Build history of the part. All positions in model axes, mm. A direction names the side the tool comes from. Round coordinates to 2 decimals unless told otherwise and drop trailing zeros. Write each loop counter-clockwise with the first axis right and the second up, starting at its lowest first coordinate (ties: lowest second). Pieces come first, ordered by that corner, then holes. Notation, with made-up numbers: (-32, 16.25) - (26, 16.25) arc R32 ccw to (26, 44.25) - close; hole circle Ø8 at (39.25, 80.25). An arc over 180 degrees is marked (long way). Write each question's results on one line, items separated by ' | '.
from build123d import *

# Parameters (mm, degrees)
EXTRUDE_1_DEPTH     = 3
SKETCH_2_W          = 40.5
SKETCH_2_H          = 13.3
SKETCH_2_W_2        = 20
SKETCH_2_H_2        = 9
SKETCH_2_W_3        = 14
SKETCH_2_H_3        = 20
SKETCH_2_W_4        = 29
SKETCH_2_H_4        = 32
CUT_EXTRUDE_1_DEPTH = 3
SKETCH_3_W          = 51.3
SKETCH_3_H          = 3
CUT_EXTRUDE_2_DEPTH = 3
SKETCH_4_W          = 4
SKETCH_4_H          = 28
SKETCH_4_W_2        = 14
SKETCH_4_H_2        = 14
EXTRUDE_2_DEPTH     = 14
CUT_EXTRUDE_3_DEPTH = 14
CUT_EXTRUDE_4_DEPTH = 14
CUT_EXTRUDE_5_DEPTH = 14
CUT_EXTRUDE_6_REACH = 216.55
SKETCH_9_R          = 2.5


with BuildPart() as part:
    # Эскиз1 → Бобышка-Вытянуть1 (new body)
    with BuildSketch(Plane(origin=(0, 0, 0), x_dir=(1, 0, 0), z_dir=(0, 1, 0))):
        Polygon((-121.424018304, 15.144551695), (-121.424018304, 41.394551695), (183.575981696, 41.394551695), (183.575981696, 15.144551695), (186.575981696, 15.144551695), (186.575981696, -11.105448305), (183.575981696, -11.105448305), (183.575981696, -37.355448305), (186.575981696, -37.355448305), (186.575981696, -63.605448305), (-118.424018304, -63.605448305), (-118.424018304, -37.355448305), (-121.424018304, -37.355448305), (-121.424018304, -11.105448305), (-118.424018304, -11.105448305), (-118.424018304, 15.144551695), align=None)
    extrude(amount=EXTRUDE_1_DEPTH)

    # Эскиз2 → Вырез-Вытянуть1 (cut)
    with BuildSketch(Plane(origin=(0, 3, 0), x_dir=(1, 0, 0), z_dir=(0, 1, 0))):
        with Locations((-58.674018304, -36.955448305)):
            Rectangle(SKETCH_2_W, SKETCH_2_H)
        with Locations((-6.874018304, -36.955448305)):
            Rectangle(SKETCH_2_W, SKETCH_2_H)
        with Locations((-6.874018304, -20.355448305)):
            Rectangle(SKETCH_2_W, SKETCH_2_H)
        with Locations((-58.674018304, -20.355448305)):
            Rectangle(SKETCH_2_W, SKETCH_2_H)
        with Locations((-6.874018304, -3.755448305)):
            Rectangle(SKETCH_2_W, SKETCH_2_H)
        with Locations((48.575981696, -1.605448305)):
            Rectangle(SKETCH_2_W_2, SKETCH_2_H_2)
        with Locations((105.575981696, -7.105448305)):
            Rectangle(SKETCH_2_W_3, SKETCH_2_H_3)
        with Locations((147.075981696, -13.105448305)):
            Rectangle(SKETCH_2_W_4, SKETCH_2_H_4)
    extrude(amount=-CUT_EXTRUDE_1_DEPTH, mode=Mode.SUBTRACT)

    # Эскиз3 → Вырез-Вытянуть2 (cut)
    with BuildSketch(Plane(origin=(0, 3, 0), x_dir=(1, 0, 0), z_dir=(0, 1, 0))):
        with Locations((-95.774018304, -62.105448305)):
            Rectangle(SKETCH_3_W, SKETCH_3_H)
        with Locations((6.825981696, -62.105448305)):
            Rectangle(SKETCH_3_W, SKETCH_3_H)
        with Locations((109.425981696, -62.105448305)):
            Rectangle(SKETCH_3_W, SKETCH_3_H)
    extrude(amount=-CUT_EXTRUDE_2_DEPTH, mode=Mode.SUBTRACT)

    # Эскиз4 → Бобышка-Вытянуть2 (add)
    with BuildSketch(Plane.XZ):
        with Locations((27.575981696, -27.394551695)):
            Rectangle(SKETCH_4_W, SKETCH_4_H)
        with Locations((-111.424018304, -34.394551695)):
            Rectangle(SKETCH_4_W_2, SKETCH_4_H_2)
        with Locations((176.575981696, -34.394551695)):
            Rectangle(SKETCH_4_W_2, SKETCH_4_H_2)
        with Locations((37.575981696, -27.394551695)):
            Rectangle(SKETCH_4_W, SKETCH_4_H)
    extrude(amount=EXTRUDE_2_DEPTH)

    # Эскиз6 → Вырез-Вытянуть3 (cut)
    with BuildSketch(Plane(origin=(39.575981696, 0, 0), x_dir=(0, 0, -1), z_dir=(1, 0, 0))):
        Polygon((13.394551695, -14), (13.394551695, 0), (38.394551695, -14), align=None)
    extrude(amount=-CUT_EXTRUDE_3_DEPTH, mode=Mode.SUBTRACT)

    # Эскиз7 → Вырез-Вытянуть4 (cut)
    with BuildSketch(Plane(origin=(183.575981696, 0, 0), x_dir=(0, 0, -1), z_dir=(1, 0, 0))):
        Polygon((27.394551695, -14), (27.394551695, 0), (38.394551695, -14), align=None)
    extrude(amount=-CUT_EXTRUDE_4_DEPTH, mode=Mode.SUBTRACT)

    # Эскиз8 → Вырез-Вытянуть5 (cut)
    with BuildSketch(Plane(origin=(-104.424018304, 0, 0), x_dir=(0, 0, -1), z_dir=(1, 0, 0))):
        Polygon((27.394551695, -14), (27.394551695, 0), (38.394551695, -14), align=None)
    extrude(amount=-CUT_EXTRUDE_5_DEPTH, mode=Mode.SUBTRACT)

    # Вырез-Вытянуть6: up to this plane
    cut_extrude_6_end = Plane(origin=(169.575981696, -14, -38.394551695), z_dir=(0, 0.6178215519319037, -0.7863183388224225))
    # Эскиз9 → Вырез-Вытянуть6 (cut, up to the surface)
    with BuildSketch(Plane(origin=(0, 0, -41.394551695), x_dir=(-1, 0, 0), z_dir=(0, 0, -1)), mode=Mode.PRIVATE) as cut_extrude_6_sk1:
        with Locations((-176.575981696, -7)):
            Circle(SKETCH_9_R)
    cut_extrude_6_tool1 = split(extrude(cut_extrude_6_sk1.sketch, amount=-CUT_EXTRUDE_6_REACH, mode=Mode.PRIVATE), bisect_by=cut_extrude_6_end, keep=Keep.BOTH, mode=Mode.PRIVATE)
    add(cut_extrude_6_tool1.solids().sort_by_distance((176.575982, -7, -41.394552))[0], mode=Mode.SUBTRACT)
    # Эскиз9 → Вырез-Вытянуть6 (cut, up to the surface)
    with BuildSketch(Plane(origin=(0, 0, -41.394551695), x_dir=(-1, 0, 0), z_dir=(0, 0, -1)), mode=Mode.PRIVATE) as cut_extrude_6_sk2:
        with Locations((111.424018304, -7)):
            Circle(SKETCH_9_R)
    cut_extrude_6_tool2 = split(extrude(cut_extrude_6_sk2.sketch, amount=-CUT_EXTRUDE_6_REACH, mode=Mode.PRIVATE), bisect_by=cut_extrude_6_end, keep=Keep.BOTH, mode=Mode.PRIVATE)
    add(cut_extrude_6_tool2.solids().sort_by_distance((-111.424018, -7, -41.394552))[0], mode=Mode.SUBTRACT)


solid = part.part
(1) Slice it at A-A, the plane z = 0. Write the cut outline in (x, y), and give its area (4 significant figures).
Worked answers:
outline: (-118.42, 0) - (-27.12, 0) - (-27.12, 3) - (-118.42, 3) - close; (13.38, 0) - (38.58, 0) - (38.58, 3) - (13.38, 3) - close; (58.58, 0) - (98.58, 0) - (98.58, 3) - (58.58, 3) - close; (112.58, 0) - (132.58, 0) - (132.58, 3) - (112.58, 3) - close; (161.58, 0) - (186.58, 0) - (186.58, 3) - (161.58, 3) - close | area: 604.5 mm2
(2) Two-plate mould, pull along X, no slides. Class faces 5 (the flat face through (-118.424, -5, -36)), 6 (the flat face through (35.576, -5, -31)), 7 (the flat face through (27.6, -6.9, -25.72)), 8 (the flat face through (183.576, -2, -34)): released by +X, released by -X, zero draft, split by the parting line, or undercut.
Worked answers:
face 5: released by -X | face 6: undercut | face 7: zero draft | face 8: released by +X
(3) Flat gauge pins, fed straight in: pin 1 Ø1.5 at (y, z) = (1, 61.5) entering from -X; pin 2 Ø7 at (y, z) = (-10, -26) entering from +X; pin 3 Ø2.5 at (y, z) = (2, 20) entering from +X. Where does each tip first touch, or does it go through?
Worked answers:
pin 1: stops at x = -70.12 | pin 2: stops at x = 39.58 | pin 3: stops at x = 183.58
(4) Tool access for faces 1 (the flat face through (-108.215, -6.902, -32.818)), 2 (the flat face through (39.576, -5, -31)), 3 (the flat face through (37.6, -6.9, -25.72)), 4 (the flat face through (179.785, -6.902, -32.818)): list every direction of +Z, -Z, +X, -X, +Y, -Y with a clear straight run to the whole face (end or side of a thin tool).
Worked answers:
face 1: +Z, -X, -Y | face 2: +Z, -Z, -Y | face 3: +Z, +X, -X, -Y | face 4: +Z, +X, -Y
(5) Slice it at C-C, the plane z = 50. Write the cut outline in (x, y).
Worked answers:
outline: (-118.42, 0) - (186.58, 0) - (186.58, 3) - (-118.42, 3) - close
(6) Slice it at D-D, the plane x = 71.5. Write the cut outline in (y, z), and give its area (3 significant figures).
Worked answers:
outline: (0, -41.39) - (3, -41.39) - (3, 63.61) - (0, 63.61) - close | area: 315 mm2
(7) Slice it at B-B, the plane x = 155. Write the cut outline in (y, z), and give its area (3 significant figures).
Worked answers:
outline: (0, -41.39) - (3, -41.39) - (3, -2.89) - (0, -2.89) - close; (0, 29.11) - (3, 29.11) - (3, 63.61) - (0, 63.61) - close | area: 219 mm2
(8) Drill centre lines: probe 1 along X at (y, z) = (-7, -36.25); probe 2 along Y at (x, z) = (104, -29); probe 3 along Z at (x, y) = (100.5, 1). Where is each one in solid material? Low to high. Write a range as [from, to].
Worked answers:
probe 1: x = [-118.42, -113.92], [-108.92, -104.42], [25.58, 29.58], [35.58, 39.58], [169.58, 174.08], [179.08, 183.58] | probe 2: y = [0, 3] | probe 3: z = [-41.39, -2.89], [17.11, 60.61]
